Could you check a few things on this model? Use its own coordinates, in mm. A direction names the side the tool comes from. Round coordinates to 2 decimals unless told otherwise and drop trailing zeros. Write each loop counter-clockwise with the first axis right and the second up, starting at its lowest first coordinate (ties: lowest second). Pieces come first, ordered by that corner, then holes. Notation, with made-up numbers: M -36.75,72 L 4.25,72 A18 cw 4.25,103 Z; hole C 15,-24 d9. An arc over 180 degrees is marked long. One line per item, written item: value. Start each with the question number.
(1) I want a section at C-C on y = -4. Please give me the cut outline in (x, z), and give its area (3 significant figures).
(2) I'm going to push flat-ended pins straight in: pin 1 Ø0.8 at (y, z) = (1.5, 6.5) entering from -X; pin 2 Ø1.4 at (y, z) = (1.5, 6.5) entering from +X. Where does each tip first touch, or does it pass through?
(3) I want a section at D-D on z = 5.5. Please give me the cut outline in (x, y) (3 decimals).
(4) Thinking about a two-plate mould opening in X: for faces 1 (the face through (-5.05, 0, 6)), 2 (the face through (2.5, -0.8, 6.4)), 3 (the face through (6, 0, 5.05)), which applies, released by +X, released by -X, zero draft, split by the parting line, or undercut?
(5) If I drill on L1, parallel to Y at x = 0, z = 6.7 (3 decimals); L2, parallel to Z at x = -4.75, y = 0.75; L3, parallel to Z at x = -0.5, y = 0 (3 decimals), over which ranges is the centre line in solid material (lowest first)?
(6) I want a section at A-A on y = 0. Please give me the cut outline in (x, z) (3 decimals).
(7) I want a section at B-B on z = -1.75. Please give me the cut outline in (x, y).
(8) Which directions (+Z, -Z, +X, -X, +Y, -Y) give clear straight access to the entire face, cutting with the end or side of a thin tool? Please do faces 4 (the face through (5.05, 0, 6)), 5 (the face through (0, -5.05, 1)), 6 (the face through (-6, 0, 5.05)).
```python
from build123d import *

# Parameters (mm, degrees)
F1_DEPTH = 5.05
F2_R     = 2.625
F5_R     = 2.625


with BuildPart() as f1:
    # F0 (on Front) → F1 (new body, symmetric)
    with BuildSketch(Plane.XZ):
        Polygon((0, 7.75), (-5.05, 7.75), (-5.05, 5.05), (-7.75, 5.05), (-7.75, 0), (-7.75, -5.05), (7.75, -5.05), (7.75, 0), (7.75, 5.05), (5.05, 5.05), (5.05, 7.75), align=None)
    extrude(amount=F1_DEPTH, both=True)

    # F4: sweep along a path in F3
    with BuildLine(Plane.XZ) as f4_path:
        Line((-10.5985039845, 0), (11.5115959197, 0))
    # F2 (on Right) → F4 (sweep, cut)
    with BuildSketch(Plane.YZ):
        Circle(F2_R)
    sweep(path=f4_path.line, mode=Mode.SUBTRACT)

    # F7: sweep along a path in F6
    with BuildLine(Plane.XZ) as f7_path:
        Line((0, 10.9545877203), (0, 5))
        ThreePointArc((0, 5), (1.4644660941, 1.4644660941), (5, 0))
    # F5 (on face) → F7 (sweep, cut)
    with BuildSketch(Plane.XY.offset(7.75)):
        Circle(F5_R)
    sweep(path=f7_path.line, mode=Mode.SUBTRACT)

    # F8: sweep along a path in F6
    with BuildLine(Plane.XZ) as f8_path:
        Line((0, 10.9545877203), (0, 5))
        ThreePointArc((0, 5), (-1.4644660941, 1.4644660941), (-5, 0))
    # F5 (on face) → F8 (sweep, cut)
    with BuildSketch(Plane.XY.offset(7.75)):
        Circle(F5_R)
    sweep(path=f8_path.line, mode=Mode.SUBTRACT)


solid = f1.part
```
Found:
1. outline: M -7.75,-5.05 L 7.75,-5.05 L 7.75,5.05 L 5.05,5.05 L 5.05,7.75 L -5.05,7.75 L -5.05,5.05 L -7.75,5.05 Z
1. area: 184 mm²
2. pin 1: stops at x = -5.05
2. pin 2: stops at x = 5.05
3. outline: M -5.05,-5.05 L 5.05,-5.05 L 5.05,5.05 L -5.05,5.05 Z; hole C 0,0 d5.25
4. face 1: released by -X
4. face 2: undercut
4. face 3: zero draft
5. L1: y = -5.05 to -2.625, 2.625 to 5.05
5. L2: z = -5.05 to -2.52, 2.53 to 7.75
5. L3: z = -5.05 to -2.625
6. outline: M -7.75,-5.05 L 7.75,-5.05 L 7.75,-2.625 L -7.75,-2.625 Z; M -7.75,2.625 L -5,2.625 A2.375 ccw -2.625,5 L -2.625,7.75 L -5.05,7.75 L -5.05,5.05 L -7.75,5.05 Z; M 2.625,5 A2.375 ccw 5,2.625 L 7.75,2.625 L 7.75,5.05 L 5.05,5.05 L 5.05,7.75 L 2.625,7.75 Z
7. outline: M -7.75,-5.05 L 7.75,-5.05 L 7.75,-1.96 L -7.75,-1.96 Z; M -7.75,1.96 L 7.75,1.96 L 7.75,5.05 L -7.75,5.05 Z
8. face 4: +Z, +X, +Y, -Y
8. face 5: +Z, -Z, +X, -X, -Y
8. face 6: +Z, -X, +Y, -Y
